Geometry check sheet. Reference: the model listing, model coordinates, mm. Face numbers are marked on the shaded views. A direction names the side the tool comes from. Coordinates: 2 decimals unless noted, no trailing zeros. Write each loop counter-clockwise with the first axis right and the second up, starting at its lowest first coordinate (ties: lowest second). Pieces come first, ordered by that corner, then holes. Notation, with made-up numbers: (41, -21.75) - (57, -21.75) arc R30 ccw to (57, 5.25) - close; hole circle Ø2 at (-39.5, 58). An arc over 180 degrees is marked (long way). Answer as a JSON object with one key per item and string values. Group by question number.
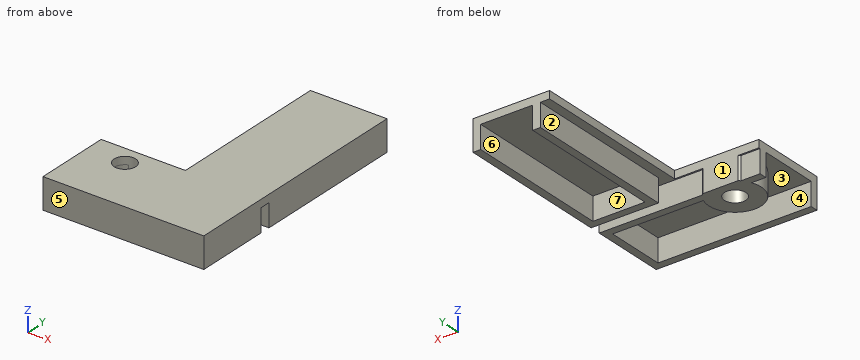
from build123d import *

# Parameters (mm, degrees)
CYLINDER005_R     = 1.4
CYLINDER005_DEPTH = 10
EXTRUDE001_DEPTH  = 3
SKETCH002_R       = 1.4
EXTRUDE002_DEPTH  = 4
EXTRUDE_DEPTH     = 1


with BuildPart() as cylinder005:
    # Cylinder005 → Cylinder005 (new body)
    with BuildSketch(Plane(origin=(-5, 2.5, -5), x_dir=(1, 0, 0), z_dir=(0, 0, 1))):
        Circle(CYLINDER005_R)
    extrude(amount=CYLINDER005_DEPTH)


with BuildPart() as extrude001:
    # Sketch001 → Extrude001 (new body)
    with BuildSketch(Plane.XY.offset(10)):
        Polygon((-21, 10), (0, 10), (0, 9), (-20, 9), (-20, 1.2), (0, 1.2), (0, 0.2), (-21, 0.2), align=None)
        Polygon((-21, -1.2), (-12.2, -1.2), (-12.2, -21.5), (-13.2, -21.5), (-13.2, -2.2), (-20, -2.2), (-20, -21.5), (-21, -21.5), align=None)
    extrude(amount=-EXTRUDE001_DEPTH)


with BuildPart() as extrude001_1:
    # Extrude001 placement: moved
    add(extrude001.part.moved(Location((0, 0, -8))))


with BuildPart() as extrude002:
    # Sketch002 → Extrude002 (new body)
    with BuildSketch(Plane.XY.offset(10)):
        with BuildLine():
            ThreePointArc((-2.695656, 0), (-5, 5.9), (-7.304344, 0))
            Line((-7.304344, 0), (-2.695656, 0))
        make_face()
        with Locations((-5, 2.5)):
            Circle(SKETCH002_R, mode=Mode.SUBTRACT)
    extrude(amount=-EXTRUDE002_DEPTH)


with BuildPart() as extrude002_1:
    # Extrude002 placement: moved
    add(extrude002.part.moved(Location((0, 0, -7))))


with BuildPart() as body001:
    # Sketch → Extrude (new body)
    with BuildSketch(Plane.XY):
        Polygon((-11, 0), (0, 0), (0, 10), (-21, 10), (-21, -21.5), (-11, -21.5), align=None)
    extrude(amount=EXTRUDE_DEPTH)


with BuildPart() as body001_1:
    # Extrude placement: moved
    add(body001.part.moved(Location((0, 0, 2))))

    # Fusion012: union Extrude001, Extrude002
    add(extrude001_1.part)
    add(extrude002_1.part)

    # Cut001: cut Cylinder005
    add(cylinder005.part, mode=Mode.SUBTRACT)


with BuildPart() as body003:
    # Part__Mirroring002: instance of Body001
    add(body001_1.part.mirror(Plane(origin=(0, -21.5, 0), x_dir=(1, 0, 0), z_dir=(0, 1, 0))))


with BuildPart() as part_mirroring004:
    # Part__Mirroring004: instance of Body003
    add(body003.part.mirror(Plane(origin=(0, -21.5, 0), x_dir=(0, -1, 0), z_dir=(1, 0, 0))))


solid = part_mirroring004.part
(1) Draft check along Y on the marked faces 4, 5, 6 and 7. Enter one of: +Y half, -Y half, draft (parallel to the pull), parting line (faces both ways), or undercut.
(2) Material ranges on L1, parallel to Y at x = 19.75, z = 1.95; L2, parallel to Y at x = 5, z = -0.1; L3, parallel to X at y = -37.5, z = 0.3, recorded low to high. Write a range as [from, to].
(3) Section check C-C (y = -51). Record the cut outline in (x, z).
(4) Section check A-A (z = 1.05). Record the cut outline in (x, y), and give its area (3 significant figures).
(5) Section check B-B (x = 5). Record the cut outline in (y, z).
(6) Set-up check for the marked faces 1, 2 and 3: record each of +Z, -Z, +X, -X, +Y, -Y from which the full face is reachable in a straight line by a thin tool's end or side.
(7) Gauge pin test, flat ends, axial feed: pin 1 (4 mm diameter, centred on x = 7.5, y = -39, fed in from -Z); pin 2 (1.5 mm diameter, centred on x = 17, z = 0, fed in from +Y); pin 3 (0.9 mm diameter, centred on y = -35.5, z = 0.5, fed in from -X); pin 4 (0.7 mm diameter, centred on x = 1, z = 1, fed in from +Y). Record the tip position at first contact, or that the pin passes through.
(8) Section check D-D (x = 14). Record the cut outline in (y, z).
Conclusion:
{
 "1": {"face 4": "undercut", "face 5": "-Y half", "face 6": "draft", "face 7": "+Y half"},
 "2": {"L1": "y = [-53, -52], [-44.2, -43.2], [-41.8, -40.8]", "L2": "y = [-53, -52], [-48.9, -46.9], [-44.1, -43]", "L3": "x = [12.2, 13.2], [20, 21]"},
 "3": {"outline": "(0, 2) - (20, 2) - (20, -1) - (21, -1) - (21, 3) - (0, 3) - close"},
 "4": {"outline": "(0, -53) - (21, -53) - (21, -43.2) - (7.5, -43.2) arc R3.4 ccw to (7.3, -43) - (2.7, -43) arc R3.4 ccw to (2.5, -43.2) - (0, -43.2) - (0, -44.2) - (1.86, -44.2) arc R3.4 ccw (long way) to (8.14, -44.2) - (20, -44.2) - (20, -52) - (0, -52) - close; (12.2, -41.8) - (21, -41.8) - (21, -21.5) - (20, -21.5) - (20, -40.8) - (13.2, -40.8) - (13.2, -21.5) - (12.2, -21.5) - close; hole circle Ø2.8 at (5, -45.5)", "area": "119 mm^2"},
 "5": {"outline": "(-53, -1) - (-52, -1) - (-52, 2) - (-48.9, 2) - (-48.9, -1) - (-46.9, -1) - (-46.9, 3) - (-53, 3) - close; (-44.1, -1) - (-43, -1) - (-43, 3) - (-44.1, 3) - close"},
 "6": {"face 1": "+Z, -Z, -X, +Y", "face 2": "-Z, -X, +Y", "face 3": "-Z"},
 "7": {"pin 1": "passes through", "pin 2": "stops at y = -40.8", "pin 3": "stops at x = 12.2", "pin 4": "stops at y = -43.2"},
 "8": {"outline": "(-53, -1) - (-52, -1) - (-52, 2) - (-44.2, 2) - (-44.2, -1) - (-43.2, -1) - (-43.2, 2) - (-41.8, 2) - (-41.8, -1) - (-40.8, -1) - (-40.8, 2) - (-21.5, 2) - (-21.5, 3) - (-53, 3) - close"}
}
